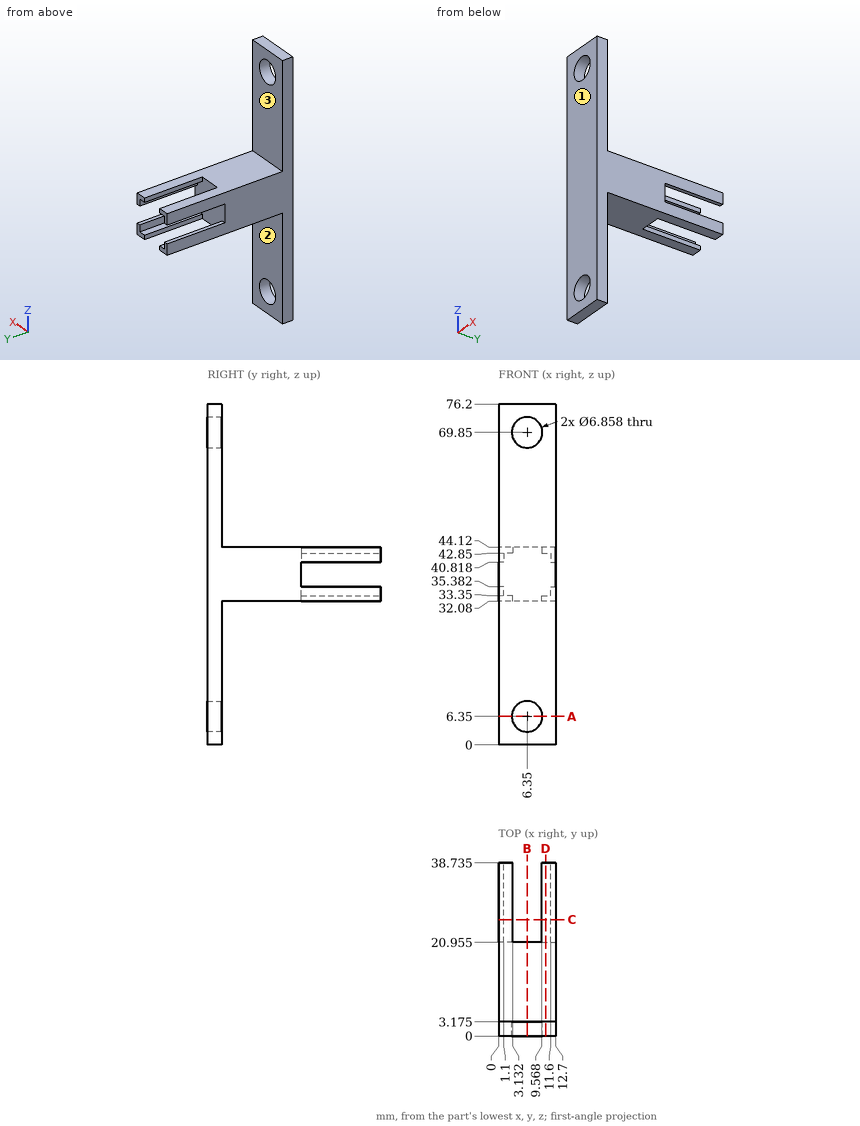
The figure shows three views and two pictorial views of one solid part (mm, origin at its lowest corner). Answer the questions. A direction names the side the tool comes from. Coordinates: 2 decimals unless noted, no trailing zeros. Order: outer loops, then holes, each group sorted by start corner. A loop starts at its lowest first (then second) coordinate and runs counter-clockwise, first axis right, second up. Notation, with made-up numbers: (49, 15.5) - (100, 15.5) arc R28 ccw to (100, 34.5) - close; hole circle Ø6 at (39.5, -17.75). An arc over 180 degrees is marked (long way). Answer as a JSON object with one key per item and string values.
1. A tool of negligible diameter and unlimited length cuts with its end or side. For the marked faces 1, 2 and 3, from which of +Z, -Z, +X, -X, +Y, -Y can it reach the whole face along a straight path? Write none if from no direction.
Output values:
{"face 1": "+Z, -Z, +X, -X, -Y", "face 2": "-Z, +X, -X, +Y", "face 3": "+Z, +X, -X, +Y"}
2. Find section C-C on y = 26. Determine the outline of the cut face in (x, z).
Output values:
{"outline": "(0, 32.08) - (3.13, 32.08) - (3.13, 33.35) - (1.1, 33.35) - (1.1, 35.38) - (0, 35.38) - close; (0, 40.82) - (1.1, 40.82) - (1.1, 42.85) - (3.13, 42.85) - (3.13, 44.12) - (0, 44.12) - close; (9.57, 32.08) - (12.7, 32.08) - (12.7, 35.38) - (11.6, 35.38) - (11.6, 33.35) - (9.57, 33.35) - close; (9.57, 42.85) - (11.6, 42.85) - (11.6, 40.82) - (12.7, 40.82) - (12.7, 44.12) - (9.57, 44.12) - close"}
3. Each of these flat-tipped pins is pushed along its axis until it touches: P1, Ø0.5, axis at x = 0.5, y = 34, coming from the -Z side; P2, Ø1, axis at x = 10.5, y = 30.5, coming from the +Z side; P3, Ø4, axis at x = 4.5, z = 12.5, coming from the +Y side (3 decimals). Where does it stop, or does it pass through?
Output values:
{"P1": "stops at z = 32.08", "P2": "stops at z = 44.12", "P3": "stops at y = 3.175"}
4. Consider line 1 (Z direction, x = 10.25, y = 37); line 2 (X direction, y = 1, z = 6); line 3 (Z direction, x = 3.75, y = 4). Determine where each line is inside the solid, lowest interval first.
Output values:
{"line 1": "z = 32.08 to 33.35, 42.85 to 44.12", "line 2": "x = 0 to 2.94, 9.76 to 12.7", "line 3": "z = 32.08 to 44.12"}
5. Find section D-D on x = 10.5. Determine the outline of the cut face in (y, z) (3 decimals), plus the area to 3 significant figures.
Output values:
{"outline": "(0, 0) - (3.175, 0) - (3.175, 32.08) - (38.735, 32.08) - (38.735, 33.35) - (20.955, 33.35) - (20.955, 42.85) - (38.735, 42.85) - (38.735, 44.12) - (3.175, 44.12) - (3.175, 76.2) - (0, 76.2) - close", "area": "501 mm²"}
6. Find section A-A on z = 6.35. Determine the outline of the cut face in (x, y) (3 decimals), plus the area to 3 significant figures.
Output values:
{"outline": "(0, 0) - (2.921, 0) - (2.921, 3.175) - (0, 3.175) - close; (9.779, 0) - (12.7, 0) - (12.7, 3.175) - (9.779, 3.175) - close", "area": "18.5 mm²"}
7. Find section B-B on x = 6.35. Determine the outline of the cut face in (y, z) (3 decimals), plus the area to 3 significant figures.
Output values:
{"outline": "(0, 0) - (3.175, 0) - (3.175, 2.921) - (0, 2.921) - close; (0, 9.779) - (3.175, 9.779) - (3.175, 32.08) - (20.955, 32.08) - (20.955, 44.12) - (3.175, 44.12) - (3.175, 66.421) - (0, 66.421) - close; (0, 73.279) - (3.175, 73.279) - (3.175, 76.2) - (0, 76.2) - close", "area": "412 mm²"}
